```python
from build123d import *

# Parameters (mm, degrees)
SZKIC1_W                    = 35
SZKIC1_H                    = 40
DODANIE_WYCI_GNI_CIE1_DEPTH = 980
SZKIC2_W                    = 100
SZKIC2_H                    = 40
DODANIE_WYCI_GNI_CIE2_DEPTH = 10
SZKIC3_W                    = 25
SZKIC3_H                    = 40
DODANIE_WYCI_GNI_CIE3_DEPTH = 50
SZKIC4_R                    = 10
WYTNIJ_WYCI_GNI_CIE3_DEPTH  = 1060.811303959


with BuildPart() as part:
    # Szkic1 → Dodanie-wyciągnięcie1 (new body)
    with BuildSketch(Plane.XY):
        with Locations((17.5, 20)):
            Rectangle(SZKIC1_W, SZKIC1_H)
    extrude(amount=DODANIE_WYCI_GNI_CIE1_DEPTH)

    # Szkic2 → Dodanie-wyciągnięcie2 (add)
    with BuildSketch(Plane.XY.offset(980)):
        with Locations((17.5, 20)):
            Rectangle(SZKIC2_W, SZKIC2_H)
    dodanie_wyci_gni_cie2 = extrude(amount=DODANIE_WYCI_GNI_CIE2_DEPTH)

    # Szkic3 → Dodanie-wyciągnięcie3 (add)
    with BuildSketch(Plane.XY.offset(990)):
        with Locations((-20, 20)):
            Rectangle(SZKIC3_W, SZKIC3_H)
        with Locations((55, 20)):
            Rectangle(SZKIC3_W, SZKIC3_H)
    dodanie_wyci_gni_cie3 = extrude(amount=DODANIE_WYCI_GNI_CIE3_DEPTH)

    # Szkic4 → Wytnij-wyciągnięcie3 (cut, through all)
    with BuildSketch(Plane(origin=(167.5, 0, 0), x_dir=(0, 0, -1), z_dir=(1, 0, 0))):
        with Locations((-1020, 20)):
            Circle(SZKIC4_R)
    wytnij_wyci_gni_cie3 = extrude(amount=-WYTNIJ_WYCI_GNI_CIE3_DEPTH, mode=Mode.SUBTRACT)

    # Lustro1: Dodanie-wyciągnięcie2, Dodanie-wyciągnięcie3, Wytnij-wyciągnięcie3 across plane
    add(dodanie_wyci_gni_cie2.mirror(Plane(origin=(0, 0, 490), x_dir=(1, 0, 0), z_dir=(0, 0, -1))))
    add(dodanie_wyci_gni_cie3.mirror(Plane(origin=(0, 0, 490), x_dir=(1, 0, 0), z_dir=(0, 0, -1))))
    add(wytnij_wyci_gni_cie3.mirror(Plane(origin=(0, 0, 490), x_dir=(1, 0, 0), z_dir=(0, 0, -1))), mode=Mode.SUBTRACT)


solid = part.part
```
Can you work these out from the model? Positions are in its coordinate system, mm. A direction names the side the tool comes from. Give positions to 0.01 mm unless a question says otherwise; leave off trailing zeros. Loops run counter-clockwise (first coordinate to the right, second up) from the corner with the lowest first, then second, coordinate; pieces in that order, holes last. Notation, with made-up numbers: M 13,-38 L 30,-38 A8 ccw 30,-32 Z; hole C 59,-16.75 d10. An arc over 180 degrees is marked long. One line per question, with ' | ' between items. Start each with the question number.
Q1. If we section it at B-B (z = -40): Please give me the cut outline in (x, y), plus the area to 3 significant figures.
Q2. If we section it at C-C (y = 20): State how many separate pieces and enclosed holes the cut face has, plus the area to 3 significant figures.
Q3. If I drill on line 1 (Y direction, x = -27, z = -40); line 2 (Z direction, x = 53, y = 6); line 3 (Z direction, x = 18.5, y = 11.5), over which ranges is the centre line in solid material (lowest first)? Write a range as from..to.
Q4. If we mould it in two halves opening along Y, with no side actions, what happens to faces 1 (the cylindrical face through (55.18, 23, 1010.46)), 2 (the flat face through (17, 40, 620)), 3 (the flat face through (42.5, 20, 1009))? For each: +Y half, -Y half, draft (parallel to the pull), parting line (faces both ways), or undercut.
Q5. For faces 4 (the flat face through (35, 20, 483)), 5 (the flat face through (17, 20, -10)), 6 (the flat face through (-7.5, 20, 1009)), 7 (the flat face through (0, 20, 483)), which set-ups out of +Z, -Z, +X, -X, +Y, -Y let a thin tool reach every point of the face, with its end or its side?
Q6. If we section it at A-A (x = -23.5): Please give me the cut outline in (y, z), plus the area to 3 significant figures.
Q7. For pin 1 Ø1 at (x, y) = (-0.5, 30.5) entering from -Z; pin 2 Ø10 at (y, z) = (11.5, 238.5) entering from +X; pin 3 Ø12 at (y, z) = (20, -40) entering from +X; pin 4 Ø20 at (x, y) = (26.5, 21.5) entering from +Z, each with a flat end and sliding along its axis, tell me the tip position at first contact or that it passes through.
Q8. If we section it at D-D (z = 439): Please give me the cut outline in (x, y), plus the area to 3 significant figures.
Computed:
1) outline: M -32.5,0 L -7.5,0 L -7.5,10 L -32.5,10 Z; M -32.5,30 L -7.5,30 L -7.5,40 L -32.5,40 Z; M 42.5,0 L 67.5,0 L 67.5,10 L 42.5,10 Z; M 42.5,30 L 67.5,30 L 67.5,40 L 42.5,40 Z | area: 1,000 mm²
2) separate pieces: 5 | enclosed holes: 0 | area: 39,300 mm²
3) line 1: y = 0..10, 30..40 | line 2: z = -60..0, 980..1040 | line 3: z = -10..990
4) face 1: undercut | face 2: +Y half | face 3: draft
5) face 4: +X, +Y, -Y | face 5: -Z, +Y, -Y | face 6: +Z, +Y, -Y | face 7: -X, +Y, -Y
6) outline: M 0,-60 L 40,-60 L 40,0 L 0,0 Z; M 0,980 L 40,980 L 40,1040 L 0,1040 Z; hole C 20,-40 d20; hole C 20,1020 d20 | area: 4,170 mm²
7) pin 1: stops at z = -10 | pin 2: stops at x = 35 | pin 3: passes through | pin 4: stops at z = 990
8) outline: M 0,0 L 35,0 L 35,40 L 0,40 Z | area: 1,400 mm²
